Verification items for the finished model (mm, model axes). A direction names the side the tool comes from. Coordinates: 2 decimals unless noted, no trailing zeros. Write each loop counter-clockwise with the first axis right and the second up, starting at its lowest first coordinate (ties: lowest second). Pieces come first, ordered by that corner, then holes. Notation, with made-up numbers: M 74,72 L 111,72 A20 cw 111,101 Z; hole C 29.5,-20 d2. An arc over 180 degrees is marked long. Answer in a Markdown table with one row per item.
from build123d import *

# Parameters (mm, degrees)
F0_R     = 7
F0_R_2   = 4.4
F1_DEPTH = 2.5
F0_R_3   = 3.5
F2_DEPTH = 9.2
F3_DEPTH = 4.2


with BuildPart() as f1:
    # F0 (on Top) → F1 (new body)
    with BuildSketch(Plane.XY):
        Circle(F0_R)
        Circle(F0_R_2, mode=Mode.SUBTRACT)
    extrude(amount=F1_DEPTH)

    # F0 (on Top) → F2 (join)
    with BuildSketch(Plane.XY):
        Circle(F0_R_2)
        Circle(F0_R_3, mode=Mode.SUBTRACT)
    extrude(amount=F2_DEPTH)

    # F0 (on Top) → F3 (join)
    with BuildSketch(Plane.XY):
        Circle(F0_R_3)
    extrude(amount=F3_DEPTH)


solid = f1.part
1) Release check for a two-part mould opening along X. For faces 1 (the face through (0, -5, 2.5)), 2 (the face through (4.197, 1.322, 5.803)), 3 (the face through (3.233, -1.341, 6.665)) record: +X half, -X half, draft (parallel to the pull), parting line (faces both ways), or undercut.
Response values:
| item | result |
|---|---|
| face 1 | draft |
| face 2 | parting line |
| face 3 | undercut |
2) Depth check by flat-ended pin: pin 1 (1.5 mm diameter, centred on x = 2.5, z = 2, fed in from -Y); pin 2 (1.5 mm diameter, centred on y = 1, z = 3.5, fed in from -X). Enter the tip coordinate at first touch or a pass-through.
Response values:
| item | result |
|---|---|
| pin 1 | stops at y = -6.78 |
| pin 2 | stops at x = -4.39 |
3) Sectioned sample at C-C (z = 1.5). Record the cut outline in (x, y), then the cut area to 3 significant figures.
Response values:
| item | result |
|---|---|
| outline | C 0,0 d14 |
| area | 154 mm² |
4) Sectioned sample at D-D (z = 4). Record the cut outline in (x, y).
Response values:
| item | result |
|---|---|
| outline | C 0,0 d8.8 |
5) Sectioned sample at A-A (x = 0). Record the cut outline in (y, z).
Response values:
| item | result |
|---|---|
| outline | M -7,0 L 7,0 L 7,2.5 L 4.4,2.5 L 4.4,9.2 L 3.5,9.2 L 3.5,4.2 L -3.5,4.2 L -3.5,9.2 L -4.4,9.2 L -4.4,2.5 L -7,2.5 Z |
6) Thickness scan on L1, parallel to Y at x = 0, z = 6.65; L2, parallel to Z at x = -4.25, y = -1.5; L3, parallel to Z at x = -0.75, y = 0. Record the ranges inside material, lowest first. Write a range as [from, to].
Response values:
| item | result |
|---|---|
| L1 | y = [-4.4, -3.5], [3.5, 4.4] |
| L2 | z = [0, 2.5] |
| L3 | z = [0, 4.2] |
7) Tool access check on faces 4 (the face through (0, -4, 9.2)), 5 (the face through (0, 0, 4.2)). Record the directions out of +Z, -Z, +X, -X, +Y, -Y that give a thin tool (end or side, any length) a straight path to the whole face; none if there is none.
Response values:
| item | result |
|---|---|
| face 4 | +Z, +X, -X, +Y, -Y |
| face 5 | +Z |
